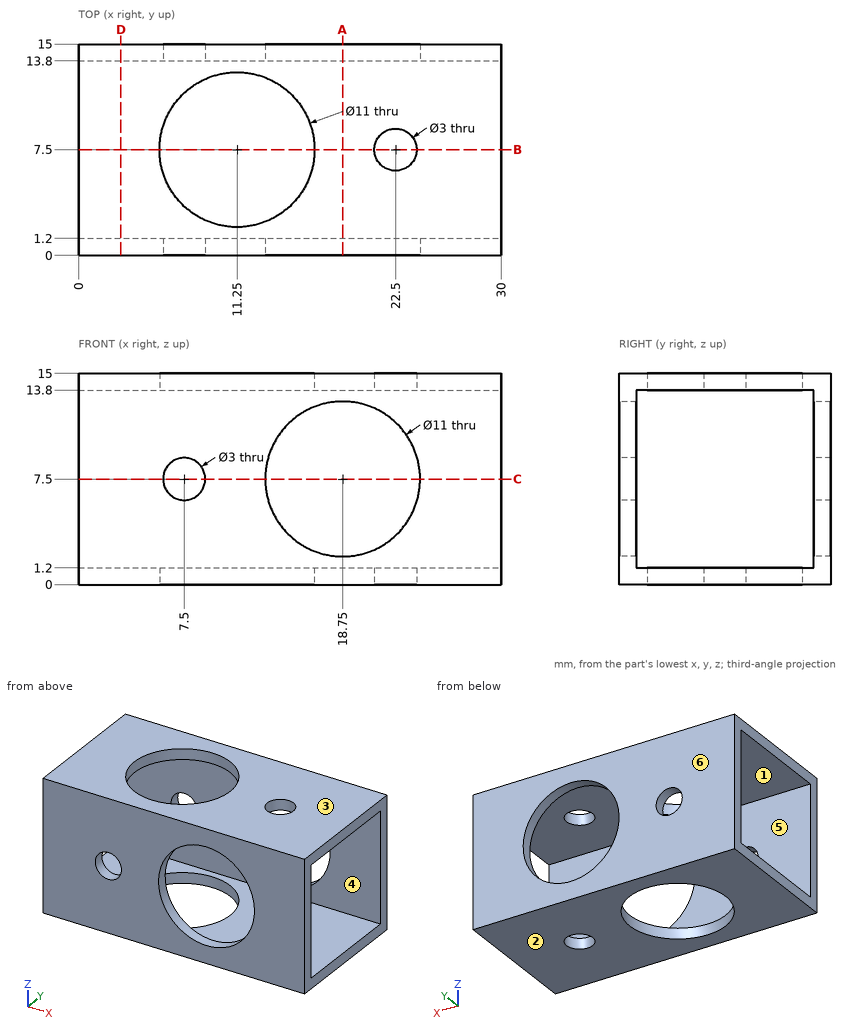
For this review, use the dimensioned drawing (mm, ordinates from the lowest corner) and the shaded views. A direction names the side the tool comes from. Coordinates: 2 decimals unless noted, no trailing zeros. Write each loop counter-clockwise with the first axis right and the second up, starting at its lowest first coordinate (ties: lowest second). Pieces come first, ordered by that corner, then holes. Notation, with made-up numbers: (30, 59) - (53, 59) arc R29 ccw to (53, 92) - close; hole circle Ø6 at (69, 14.25). An arc over 180 degrees is marked (long way). Answer in a Markdown table with one row per item. Add a question column.
Q1. To check wall thickness, follow line 1 along X through (y, z) = (0.9, 7.5); line 2 along X through (y, z) = (7.5, 0.4); line 3 along Z through (x, y) = (4.5, 6). State the ranges of each line that lie inside material, in increasing order. Write a range as from..to.
Q2. Consider section C-C on z = 7.5. Give the boundary of the cut face in (x, y).
Q3. Consider section B-B on y = 7.5. Give the boundary of the cut face in (x, z).
Q4. Consider section D-D on x = 3. Give the boundary of the cut face in (y, z).
Q5. For the marked faces 1 and 2, list the 3-axis set-ups (+Z, -Z, +X, -X, +Y, -Y) from which the entire face can be reached by the end or side of a thin tool; tool diameter is ignored.
Q6. Clearance check with a flat-ended pin moving along its axis: pin 1 (6.5 mm diameter, centred on x = 11.25, y = 7.5, fed in from +Z). State where the tip first meets the part, or that it passes through.
Q7. Draft analysis for pull direction Y (two halves, no side actions). For the marked faces 3, 4, 5 and 6, state which applies: +Y half, -Y half, draft (parallel to the pull), parting line (faces both ways), or undercut.
Q8. Consider section A-A on x = 18.75. Give the boundary of the cut face in (y, z), then the cut area to 3 significant figures.
Answers below:
| question | item | result |
|---|---|---|
| 1 | line 1 | 0..6, 9..13.25, 24.25..30 |
| 1 | line 2 | 0..5.75, 16.75..21, 24..30 |
| 1 | line 3 | 0..1.2, 13.8..15 |
| 2 | outline | (0, 0) - (6, 0) - (6, 1.2) - (0, 1.2) - close; (0, 13.8) - (6, 13.8) - (6, 15) - (0, 15) - close; (9, 0) - (13.25, 0) - (13.25, 1.2) - (9, 1.2) - close; (9, 13.8) - (13.25, 13.8) - (13.25, 15) - (9, 15) - close; (24.25, 0) - (30, 0) - (30, 1.2) - (24.25, 1.2) - close; (24.25, 13.8) - (30, 13.8) - (30, 15) - (24.25, 15) - close |
| 3 | outline | (0, 0) - (5.75, 0) - (5.75, 1.2) - (0, 1.2) - close; (0, 13.8) - (5.75, 13.8) - (5.75, 15) - (0, 15) - close; (16.75, 0) - (21, 0) - (21, 1.2) - (16.75, 1.2) - close; (16.75, 13.8) - (21, 13.8) - (21, 15) - (16.75, 15) - close; (24, 0) - (30, 0) - (30, 1.2) - (24, 1.2) - close; (24, 13.8) - (30, 13.8) - (30, 15) - (24, 15) - close |
| 4 | outline | (0, 0) - (15, 0) - (15, 15) - (0, 15) - close; hole (1.2, 1.2) - (13.8, 1.2) - (13.8, 13.8) - (1.2, 13.8) - close |
| 5 | face 1 | +X, -X |
| 5 | face 2 | -Z, +X, -X, +Y, -Y |
| 6 | pin 1 | through |
| 7 | face 3 | draft |
| 7 | face 4 | undercut |
| 7 | face 5 | undercut |
| 7 | face 6 | +Y half |
| 8 | outline | (0, 0) - (15, 0) - (15, 2) - (13.8, 2) - (13.8, 1.2) - (1.2, 1.2) - (1.2, 2) - (0, 2) - close; (0, 13) - (1.2, 13) - (1.2, 13.8) - (13.8, 13.8) - (13.8, 13) - (15, 13) - (15, 15) - (0, 15) - close |
| 8 | area | 39.8 mm² |
